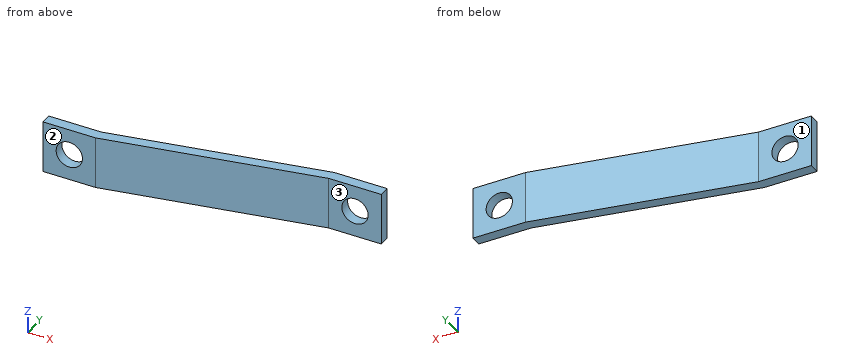
Autodesk Inventor part; units mm, degrees
ref_plane "YZ Plane" through (0, 0, 0) normal (1, 0, 0) x (0, 1, 0)
ref_plane "XZ Plane" through (0, 0, 0) normal (0, 1, 0) x (-1, 0, 0)
ref_plane "XY Plane" through (0, 0, 0) normal (0, 0, 1) x (1, 0, 0)
sketch "Szkic1" plane through (0, 0, 0) normal (0, 0, 1) x (1, 0, 0)
  line L0 (-35.4869, -5) -> (-25.4869, -5)
  line L1 (-25.4869, -3) -> (-35.4869, -3)
  line L2 (-35.4869, -5) -> (-35.4869, -3)
  line L3 (24.5131, 5) -> (14.5131, 5)
  line L4 (24.5131, 3) -> (24.5131, 3)
  line L5 (24.5131, 3) -> (24.5131, 5)
  line L6 (24.5131, 3) -> (14.5131, 3)
  line L7 (14.5131, 3) -> (-25.4869, -5)
  line L8 (-25.4869, -3) -> (14.5131, 5)
  point P0 (24.5131, 5)
  dimension "d9" = 10
  dimension "d10" = 2
  dimension "d11" = 10
  dimension "d14" = 60
  dimension "d15" = 10
extrude "Wyciągnięcie proste1" add sketch "Szkic1" along normal blind 10
sketch "Szkic2" plane through (-35.4869, -3, 0) normal (0, 1, 0) x (1, 0, 0)
  line L0 (10, 0) -> (10, -10)
  line L1 (10, -5) -> (0, -5)
  line L2 (0, 0) -> (0, -10)
  circle A0 centre (5, -5) radius 2.5
  point P0 (35.4869, 0)
  dimension "d16" = 5
extrude "Wyciągnięcie proste2" cut sketch "Szkic2" against normal blind 10
sketch "Szkic3" plane through (14.5131, 5, 0) normal (0, 1, 0) x (1, 0, 0)
  line L0 (10, 0) -> (10, -10)
  line L1 (10, -5) -> (0, -5)
  line L2 (0, 0) -> (0, -10)
  circle A0 centre (5, -5) radius 2.5
  point P0 (-14.5131, 0)
  dimension "d19" = 5
extrude "Wyciągnięcie proste3" cut sketch "Szkic3" against normal blind 10
properties part number "Docisk_sprężynka" material "Stal, węglowa"
CAD build for the part. Positions are in the model's coordinates, mm. Face numbers are marked on the shaded views. A direction names the side the tool comes from. Coordinates: 2 decimals unless noted, no trailing zeros. Loops run counter-clockwise (first coordinate to the right, second up) from the corner with the lowest first, then second, coordinate; pieces in that order, holes last. Notation, with made-up numbers: (43, 11.25) - (58, 11.25) arc R38 cw to (58, 50.25) - close; hole circle Ø4 at (69.25, 14.5). An arc over 180 degrees is marked (long way). Use one line per item in the form item = value. Start each with the question number.
1) Flat gauge pins, fed straight in: pin 1 (4 mm diameter, centred on x = -16, z = 7.5, fed in from -Y); pin 2 (3 mm diameter, centred on x = -30.49, z = 5, fed in from +Y); pin 3 (4 mm diameter, centred on x = 12.5, z = 1.5, fed in from -Y). Where does each tip first touch, or does it go through?
2) Tool access for the marked faces 1, 2 and 3: list every direction of +Z, -Z, +X, -X, +Y, -Y with a clear straight run to the whole face (end or side of a thin tool).
3) Band-saw the part on B-B (y = 4). Give the cut face in (x, z).
4) Drill centre lines: L1, parallel to Y at x = -31.5, z = 2; L2, parallel to Z at x = 18, y = 3.5; L3, parallel to Y at x = -6.5, z = 1.75. Where is each one in solid material? Low to high. Write a range as from..to.
5) Band-saw the part on D-D (x = -16.5). Give the cut face in (y, z), and give its area (3 significant figures).
6) Band-saw the part on A-A (z = 5). Give the cut face in (x, y), and give its area (4 significant figures).
7) Band-saw the part on C-C (y = 1.5). Give the cut face in (x, z), and give its area (4 significant figures).
Check values:
q1.pin_1 = -3.5
q1.pin_2 = through
q1.pin_3 = 2.2
q2.face_1 = +Z, -Z, -X, +Y
q2.face_2 = +Z, -Z, +X, -X, -Y
q2.face_3 = +Z, -Z, +X, -Y
q3.outline = (9.51, 0) - (24.51, 0) - (24.51, 10) - (9.51, 10) - close; hole circle Ø5 at (19.51, 5)
q4.L1 = -5..-3
q4.L2 = 0..3.01, 6.99..10
q4.L3 = -1.2..0.8
q5.outline = (-3.2, 0) - (-1.2, 0) - (-1.2, 10) - (-3.2, 10) - close
q5.area = 20.0 mm2
q6.outline = (-35.49, -5) - (-32.99, -5) - (-32.99, -3) - (-35.49, -3) - close; (-27.99, -5) - (-25.49, -5) - (14.51, 3) - (17.01, 3) - (17.01, 5) - (14.51, 5) - (-25.49, -3) - (-27.99, -3) - close; (22.01, 3) - (24.51, 3) - (24.51, 5) - (22.01, 5) - close
q6.area = 100.0 mm2
q7.outline = (-2.99, 0) - (7.01, 0) - (7.01, 10) - (-2.99, 10) - close
q7.area = 100.0 mm2
